Here's how the part is built. I have some questions about the finished solid (model axes, mm). Face numbers are marked on the shaded views. A direction names the side the tool comes from. Coordinates: 2 decimals unless noted, no trailing zeros. Write each loop counter-clockwise with the first axis right and the second up, starting at its lowest first coordinate (ties: lowest second). Pieces come first, ordered by that corner, then holes.
Item 1: I'm going to push flat-ended pins straight in: P1, Ø5.5, axis at y = -1.5, z = -16, coming from the -X side; P2, Ø8, axis at x = -0.5, z = 13, coming from the -Y side; P3, Ø9.5, axis at x = 0, y = 0, coming from the -Z side; P4, Ø20, axis at x = 2.5, y = -6, coming from the +Z side. Where does each tip first touch, or does it pass through?
Item 2: Please list where these lines run through material, in increasing order: line 1 (Y direction, x = 0, z = -18); line 2 (Y direction, x = 0, z = -21.75); line 3 (Z direction, x = -1, y = -34.5).
Item 3: I want a section at A-A (y = 0). Please give me the cut outline in (x, z).
Item 4: I want a section at B-B (x = 33.5). Please give me the cut outline in (y, z), and give its area (3 significant figures).
Item 5: I want a section at C-C (z = 6.5). Please give me the cut outline in (x, y).
Item 6: For the marked faces 4, 5 and 6, which set-ups out of +Z, -Z, +X, -X, +Y, -Y let a thin tool reach every point of the face, with its end or its side?
Item 7: If we mould it in two halves opening along Y, with no side actions, what happens to the marked faces 1, 2 and 3? For each: pulls with the +Y half, pulls with the -Y half, needs draft (parallel to the pull), parting line crosses it, or undercut.
Item 8: I want a section at D-D (y = 35.5). Please give me the cut outline in (x, z).
from build123d import *

# Parameters (mm, degrees)
CROQUIS1_R              = 56
SALIENTE_EXTRUIR1_DEPTH = 23
CROQUIS2_R              = 40
CORTAR_EXTRUIR1_DEPTH   = 40.5
CROQUIS3_R              = 12.5
SALIENTE_EXTRUIR2_DEPTH = 5
CORTAR_EXTRUIR2_DEPTH   = 5
CROQUIS5_R              = 6
CORTAR_EXTRUIR3_DEPTH   = 89.950829114
CROQUIS6_R              = 12.5
CORTAR_EXTRUIR4_DEPTH   = 3


with BuildPart() as part:
    # Croquis1 → Saliente-Extruir1 (new, symmetric)
    with BuildSketch(Plane.XY):
        Circle(CROQUIS1_R)
    extrude(amount=SALIENTE_EXTRUIR1_DEPTH, both=True)

    # Croquis2 → Cortar-Extruir1 (cut)
    with BuildSketch(Plane.XY.offset(23)):
        Circle(CROQUIS2_R)
    extrude(amount=-CORTAR_EXTRUIR1_DEPTH, mode=Mode.SUBTRACT)

    # Croquis3 → Saliente-Extruir2 (add)
    with BuildSketch(Plane.XY.offset(-17.5)):
        Circle(CROQUIS3_R)
    extrude(amount=SALIENTE_EXTRUIR2_DEPTH)

    # Croquis4 → Cortar-Extruir2 (cut)
    with BuildSketch(Plane.XY.offset(-12.5)):
        Polygon((0, 9.814954576), (-8.5, 4.907477288), (-8.5, -4.907477288), (0, -9.814954576), (8.5, -4.907477288), (8.5, 4.907477288), align=None)
    extrude(amount=-CORTAR_EXTRUIR2_DEPTH, mode=Mode.SUBTRACT)

    # Croquis5 → Cortar-Extruir3 (cut, through all)
    with BuildSketch(Plane.XY.offset(-17.5)):
        Circle(CROQUIS5_R)
    extrude(amount=-CORTAR_EXTRUIR3_DEPTH, mode=Mode.SUBTRACT)

    # Croquis6 → Cortar-Extruir4 (cut)
    with BuildSketch(Plane(origin=(0, 0, -23), x_dir=(-1, 0, 0), z_dir=(0, 0, -1))):
        with Locations(Location((0, 0, 0), (0, 0, 180))):
            Circle(CROQUIS6_R)
    extrude(amount=-CORTAR_EXTRUIR4_DEPTH, mode=Mode.SUBTRACT)


solid = part.part
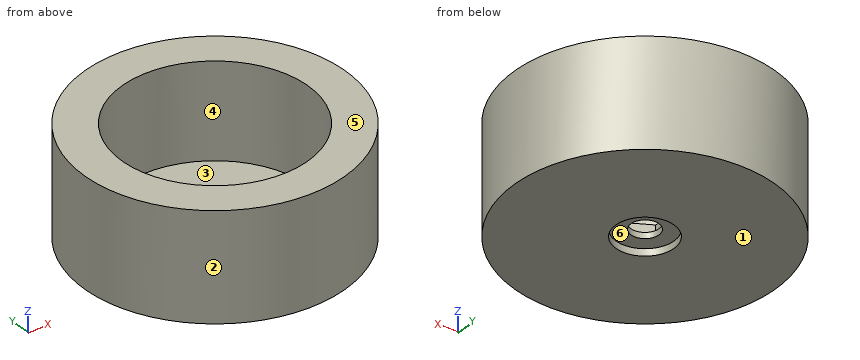
Answer:
1. P1: stops at x = -56
1. P2: stops at y = -56
1. P3: passes through
1. P4: stops at z = -12.5
2. line 1: y = -56 to -6, 6 to 56
2. line 2: y = -56 to -12.5, 12.5 to 56
2. line 3: z = -23 to -17.5
3. outline: (-56, -23) - (-12.5, -23) - (-12.5, -20) - (-6, -20) - (-6, -17.5) - (-8.5, -17.5) - (-8.5, -12.5) - (-12.5, -12.5) - (-12.5, -17.5) - (-40, -17.5) - (-40, 23) - (-56, 23) - close; (6, -20) - (12.5, -20) - (12.5, -23) - (56, -23) - (56, 23) - (40, 23) - (40, -17.5) - (12.5, -17.5) - (12.5, -12.5) - (8.5, -12.5) - (8.5, -17.5) - (6, -17.5) - close
4. outline: (-44.87, -23) - (44.87, -23) - (44.87, 23) - (21.86, 23) - (21.86, -17.5) - (-21.86, -17.5) - (-21.86, 23) - (-44.87, 23) - close
4. area: 2,360 mm2
5. outline: circle Ø112 at (0, 0); hole circle Ø80 at (0, 0)
6. face 4: +Z
6. face 5: +Z, +X, -X, +Y, -Y
6. face 6: -Z
7. face 1: needs draft
7. face 2: parting line crosses it
7. face 3: undercut
8. outline: (-43.31, -23) - (43.31, -23) - (43.31, 23) - (18.43, 23) - (18.43, -17.5) - (-18.43, -17.5) - (-18.43, 23) - (-43.31, 23) - close
